from build123d import *

# Parameters (mm, degrees)
SKETCH1_W                    = 30
SKETCH1_H                    = 60
SKETCH1_R                    = 2
BASE_FLANGE1_DEPTH           = 0.7366
EDGE_FLANGE1_STRIP_W         = 4.4196
EDGE_FLANGE1_STRIP_H         = 0.7366
EDGE_FLANGE1_STRIP_CUT_DEPTH = 30
EDGE_FLANGE1_DEPTH           = 30
EDGE_FLANGE1_PROFILE_W       = 30
EDGE_FLANGE1_PROFILE_H       = 19.2634
EDGE_FLANGE1_PROFILE_R       = 2.05
EDGE_FLANGE1_FLAT_DEPTH      = 0.7366
EDGE_FLANGE2_STRIP_W         = 4.4196
EDGE_FLANGE2_STRIP_H         = 0.7366
EDGE_FLANGE2_STRIP_CUT_DEPTH = 58.5268
EDGE_FLANGE2_DEPTH           = 58.5268
EDGE_FLANGE3_STRIP_W         = 4.4196
EDGE_FLANGE3_STRIP_H         = 0.7366
EDGE_FLANGE3_STRIP_CUT_DEPTH = 58.5268
EDGE_FLANGE3_DEPTH           = 58.5268
EDGE_FLANGE4_STRIP_W         = 4.4196
EDGE_FLANGE4_STRIP_H         = 0.7366
EDGE_FLANGE4_STRIP_CUT_DEPTH = 19.2634
EDGE_FLANGE4_DEPTH           = 19.2634
SKETCH18_R                   = 2.05
CUT_EXTRUDE1_DEPTH           = 409.590672417


# Sheet-metal steps are written as plain solids
with BuildPart() as part:
    # Sketch1 → Base-Flange1 (new body)
    with BuildSketch(Plane(origin=(0, 0, 0), x_dir=(1, 0, 0), z_dir=(0, 1, 0))):
        Rectangle(SKETCH1_W, SKETCH1_H)
        with Locations(Location((7.5, -15, 0), (0, 0, 270))):
            Circle(SKETCH1_R, mode=Mode.SUBTRACT)
        with Locations(Location((0, 15, 0), (0, 0, 270))):
            Circle(SKETCH1_R, mode=Mode.SUBTRACT)
        with Locations(Location((-7.5, -15, 0), (0, 0, 270))):
            Circle(SKETCH1_R, mode=Mode.SUBTRACT)
    extrude(amount=-BASE_FLANGE1_DEPTH)

    # Edge-Flange1 strip (across the edge) → Edge-Flange1 strip cut (cut)
    with BuildSketch(Plane(origin=(15, 0, -30), x_dir=(0, 0, 1), z_dir=(-1, 0, 0))):
        with Locations((-0.7366, -0.3683)):
            Rectangle(EDGE_FLANGE1_STRIP_W, EDGE_FLANGE1_STRIP_H)
    extrude(amount=EDGE_FLANGE1_STRIP_CUT_DEPTH, mode=Mode.SUBTRACT)

    # Edge-Flange1 bend section (across the edge) → Edge-Flange1 (add)
    with BuildSketch(Plane(origin=(15, 0, -30), x_dir=(0, 0, 1), z_dir=(-1, 0, 0))):
        with BuildLine():
            Line((0, 0.7366), (0.7366, 0.7366))
            ThreePointArc((0.7366, 0.7366), (0.952345145, 0.215745145), (1.4732, 0))
            Line((1.4732, 0), (1.4732, -0.7366))
            ThreePointArc((1.4732, -0.7366), (0.43149029, -0.30510971), (0, 0.7366))
        make_face()
    extrude(amount=EDGE_FLANGE1_DEPTH)

    # Edge-Flange1 profile (on flange) → Edge-Flange1 flat (add)
    with BuildSketch(Plane(origin=(0, 0, -30), x_dir=(-1, 0, 0), z_dir=(0, 0, -1))):
        with Locations((0, 10.3683)):
            Rectangle(EDGE_FLANGE1_PROFILE_W, EDGE_FLANGE1_PROFILE_H)
        with Locations((0, 10)):
            Circle(EDGE_FLANGE1_PROFILE_R, mode=Mode.SUBTRACT)
    extrude(amount=-EDGE_FLANGE1_FLAT_DEPTH)

    # Edge-Flange2 strip (across the edge) → Edge-Flange2 strip cut (cut)
    with BuildSketch(Plane(origin=(15, 0, 30), x_dir=(-1, 0, 0), z_dir=(0, 0, -1))):
        with Locations((-0.7366, -0.3683)):
            Rectangle(EDGE_FLANGE2_STRIP_W, EDGE_FLANGE2_STRIP_H)
    extrude(amount=EDGE_FLANGE2_STRIP_CUT_DEPTH, mode=Mode.SUBTRACT)

    # Edge-Flange2 section (across the edge) → Edge-Flange2 (add)
    with BuildSketch(Plane(origin=(15, 0, 30), x_dir=(-1, 0, 0), z_dir=(0, 0, -1))):
        with BuildLine():
            Line((0, 0.7366), (0, 19.2634))
            Line((0, 19.2634), (0.7366, 19.2634))
            Line((0.7366, 19.2634), (0.7366, 0.7366))
            ThreePointArc((0.7366, 0.7366), (0.952345145, 0.215745145), (1.4732, 0))
            Line((1.4732, 0), (1.4732, -0.7366))
            ThreePointArc((1.4732, -0.7366), (0.43149029, -0.30510971), (0, 0.7366))
        make_face()
    extrude(amount=EDGE_FLANGE2_DEPTH)

    # Edge-Flange3 strip (across the edge) → Edge-Flange3 strip cut (cut)
    with BuildSketch(Plane(origin=(-15, 0, -28.5268), x_dir=(1, 0, 0), z_dir=(0, 0, 1))):
        with Locations((-0.7366, -0.3683)):
            Rectangle(EDGE_FLANGE3_STRIP_W, EDGE_FLANGE3_STRIP_H)
    extrude(amount=EDGE_FLANGE3_STRIP_CUT_DEPTH, mode=Mode.SUBTRACT)

    # Edge-Flange3 section (across the edge) → Edge-Flange3 (add)
    with BuildSketch(Plane(origin=(-15, 0, -28.5268), x_dir=(1, 0, 0), z_dir=(0, 0, 1))):
        with BuildLine():
            Line((0, 0.7366), (0, 19.2634))
            Line((0, 19.2634), (0.7366, 19.2634))
            Line((0.7366, 19.2634), (0.7366, 0.7366))
            ThreePointArc((0.7366, 0.7366), (0.952345145, 0.215745145), (1.4732, 0))
            Line((1.4732, 0), (1.4732, -0.7366))
            ThreePointArc((1.4732, -0.7366), (0.43149029, -0.30510971), (0, 0.7366))
        make_face()
    extrude(amount=EDGE_FLANGE3_DEPTH)

    # Edge-Flange4 strip (across the edge) → Edge-Flange4 strip cut (cut)
    with BuildSketch(Plane(origin=(15, 20, -30), x_dir=(-1, 0, 0), z_dir=(0, -1, 0))):
        with Locations((-1.4732, -0.3683)):
            Rectangle(EDGE_FLANGE4_STRIP_W, EDGE_FLANGE4_STRIP_H)
    extrude(amount=EDGE_FLANGE4_STRIP_CUT_DEPTH, mode=Mode.SUBTRACT)

    # Edge-Flange4 section (across the edge) → Edge-Flange4 (add)
    with BuildSketch(Plane(origin=(15, 20, -30), x_dir=(-1, 0, 0), z_dir=(0, -1, 0))):
        with BuildLine():
            Line((-0.7366, 0.7366), (-0.7366, 68.2634))
            Line((-0.7366, 68.2634), (0, 68.2634))
            Line((0, 68.2634), (0, 0.7366))
            ThreePointArc((0, 0.7366), (0.215745145, 0.215745145), (0.7366, 0))
            Line((0.7366, 0), (0.7366, -0.7366))
            ThreePointArc((0.7366, -0.7366), (-0.30510971, -0.30510971), (-0.7366, 0.7366))
        make_face()
    extrude(amount=EDGE_FLANGE4_DEPTH)

    # Sketch18 → Cut-Extrude1 (cut, through all)
    with BuildSketch(Plane(origin=(-385, -11.740421973, -25.126127563), x_dir=(0, 0, 1), z_dir=(-1, 0, 0))):
        with Locations((-42.610472437, 21.740421973)):
            Circle(SKETCH18_R)
        with Locations((-58.610472437, 21.740421973)):
            Circle(SKETCH18_R)
        with Locations(Location((22.862727563, 21.740421973, 0), (0, 0, 90))):
            Circle(SKETCH18_R)
        with Locations(Location((38.862727563, 21.740421973, 0), (0, 0, 90))):
            Circle(SKETCH18_R)
    extrude(amount=-CUT_EXTRUDE1_DEPTH, mode=Mode.SUBTRACT)


solid = part.part
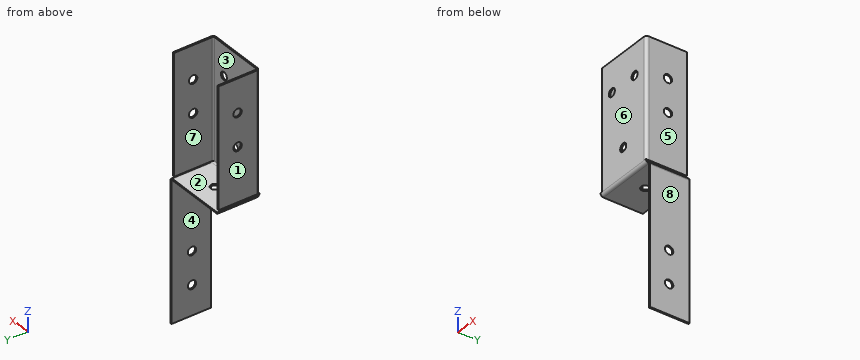
Part model, mm, in its own coordinate system. Face numbers are marked on the shaded views. A direction names the side the tool comes from. Give positions to 0.01 mm unless a question says otherwise; leave off trailing zeros. Loops run counter-clockwise (first coordinate to the right, second up) from the corner with the lowest first, then second, coordinate; pieces in that order, holes last. Notation, with made-up numbers: M 27.5,24 L 72.5,24 A14 ccw 72.5,33 Z; hole C 36.5,63.5 d2. An arc over 180 degrees is marked long. Put each result on its own line as item: value. Start each with the question number.
1) Pull direction X, two halves, no side cores. Call the marked faces 1, 2 and 3: +X half, -X half, draft (parallel to the pull), parting line (faces both ways), or undercut.
2) Probe probe 1 along Z at (x, y) = (14.45, 10); probe 2 along X at (y, z) = (5.5, -20.5); probe 3 along Z at (x, y) = (14.85, 10). List the from-to ranges inside material, lowest first.
3) Flat gauge pins, fed straight in: pin 1 (2 mm diameter, centred on x = 8, y = 16.5, fed in from +Z); pin 2 (0.8 mm diameter, centred on x = -14.5, z = -4.5, fed in from +Y); pin 3 (2.5 mm diameter, centred on y = 10, z = -2.26, fed in from +X); pin 4 (5.5 mm diameter, centred on y = 9.5, z = 15, fed in from +X). Where does each tip first touch, or does it go through?
4) Saw through at A-A (x = 7.5). List the corners of the cut face in (y, z).
5) Saw through at C-C (y = 4). List the corners of the cut face in (x, z), then the cut area to 3 significant figures.
6) Saw through at D-D (x = 0). List the corners of the cut face in (y, z).
7) 3-axis set-ups, long thin cutter, end or side, ignore diameter. For the marked faces 4, 5, 6, 7 and 8: which of +Z, -Z, +X, -X, +Y, -Y reach the whole face in a straight line?
8) Saw through at B-B (z = -15). List the corners of the cut face in (x, y), then the cut area to 3 significant figures.
Numbers:
1. face 1: -X half
1. face 2: draft
1. face 3: undercut
2. probe 1: -30.02 to -29.28, -28.53 to -4.31, -0.21 to 11.69, 15.79 to 30
2. probe 2: -15 to -14.26, 14.26 to 15
2. probe 3: -30.29 to -29.39, -28.53 to -4.31, -0.21 to 11.69, 15.79 to 30
3. pin 1: z = -29.26
3. pin 2: y = 19.26
3. pin 3: through
3. pin 4: x = 15
4. outline: M -0.74,-28.53 A1.47 ccw 0.74,-30 L 20,-30 L 20,-29.26 L 0.74,-29.26 A0.74 cw 0,-28.53 L 0,13 L -0.74,13 Z; M -0.74,17 L 0,17 L 0,30 L -0.74,30 Z
5. outline: M -15,-30 L 14.26,-30 A0.74 cw 15,-30.74 L 15,-98.26 L 15.74,-98.26 L 15.74,-30.74 A1.47 ccw 14.26,-29.26 L -15,-29.26 Z; M -15,-28.53 L -14.26,-28.53 L -14.26,30 L -15,30 Z; M 14.26,-28.53 L 15,-28.53 L 15,30 L 14.26,30 Z
5. area: 159 mm^2
6. outline: M -0.74,-28.53 A1.47 ccw 0.74,-30 L 7.95,-30 L 7.95,-29.26 L 0.74,-29.26 A0.74 cw 0,-28.53 L 0,-17 L -0.74,-17 Z; M -0.74,-13 L 0,-13 L 0,30 L -0.74,30 Z; M 12.05,-30 L 20,-30 L 20,-29.26 L 12.05,-29.26 Z
7. face 4: -Z, -X, +Y, -Y
7. face 5: +Z, +X, +Y, -Y
7. face 6: +Z, -Z, +X, -X, -Y
7. face 7: +Z, +Y
7. face 8: +Z, -Z, +X, +Y, -Y
8. outline: M -15,0.74 A1.47 ccw -13.53,-0.74 L -2,-0.74 L -2,0 L -13.53,0 A0.74 cw -14.26,0.74 L -14.26,19.26 L -15,19.26 Z; M 2,-0.74 L 13.53,-0.74 A1.47 ccw 15,0.74 L 15,19.26 L 14.26,19.26 L 14.26,0.74 A0.74 cw 13.53,0 L 2,0 Z
8. area: 46.8 mm^2
